Here's how the part is built. I have some questions about the finished solid (model axes, mm). Face numbers are marked on the shaded views. A direction names the side the tool comes from. Round coordinates to 2 decimals unless told otherwise and drop trailing zeros. Write each loop counter-clockwise with the first axis right and the second up, starting at its lowest first coordinate (ties: lowest second). Pieces come first, ordered by that corner, then holes. Notation, with made-up numbers: (87.25, 33) - (132.25, 33) arc R25 cw to (132.25, 50) - close; hole circle Ø3 at (88.5, 85.25). An arc over 180 degrees is marked (long way). One line per item, written item: value. Start each with the question number.
Item 1: Imagine slicing it at D-D, the plane x = 2. Please give me the cut outline in (y, z), then the cut area to 3 significant figures.
Item 2: Imagine slicing it at A-A, the plane z = 1.75. Count the separate pieces of the cut face and the enclosed holes in it, then the cut area to 3 significant figures.
Item 3: For the marked faces 5 and 6, which set-ups out of +Z, -Z, +X, -X, +Y, -Y let a thin tool reach every point of the face, with its end or its side?
Item 4: For P1, Ø4, axis at y = -6, z = 2.5, coming from the -X side; P2, Ø3.5, axis at x = 8.5, y = -1, coming from the -Z side, each with a flat end and sliding along its axis, tell me the tip position at first contact or that it passes through.
Item 5: Imagine slicing it at B-B, the plane x = 40. Please give me the cut outline in (y, z).
Item 6: Imagine slicing it at C-C, the plane x = -26.75. Please give me the cut outline in (y, z), then the cut area to 3 significant figures.
Item 7: Thinking about a two-plate mould opening in X: for the marked faces 1, 2, 3 and 4, which applies, released by +X, released by -X, zero draft, split by the parting line, or undercut?
Item 8: If I drill on line 1 (Y direction, x = -26.75, z = -1); line 2 (Y direction, x = 20, z = 1); line 3 (Y direction, x = 0, z = 1.25), over which ranges is the centre line in solid material (lowest first)?
```python
from build123d import *

# Parameters (mm, degrees)
F0_W        = 60
F0_H        = 15
F0_R        = 1.5
F0_W_2      = 40
F0_R_2      = 1.75
F1_DEPTH    = 5
F2_T        = -2
F3_R        = 5
F4_R        = 5
F5_T1_DEPTH = 100
F5_T3_DEPTH = 5
F5_T6_ANGLE = 90
F5_T8_ANGLE = 90


# Not quite as in the source:
# - a fillet or chamfer that OpenCascade refuses, or shapes differently, is made with other operations: its cross-section is extruded or revolved along the edge and cut away or added


with BuildPart() as f1:
    # F0 (on Top) → F1 (new body, symmetric)
    with BuildSketch(Plane.XY):
        with Locations((-20, 0)):
            Rectangle(F0_W, F0_H)
        with Locations((-45.75, 0)):
            Circle(F0_R, mode=Mode.SUBTRACT)
        with Locations((-26.75, 0)):
            Circle(F0_R, mode=Mode.SUBTRACT)
        with Locations((30, 0)):
            Rectangle(F0_W_2, F0_H)
        with Locations((20, 0)):
            Circle(F0_R_2, mode=Mode.SUBTRACT)
        with Locations((40, 0)):
            Circle(F0_R_2, mode=Mode.SUBTRACT)
    extrude(amount=F1_DEPTH, both=True)

    # F2
    f2_openings = [f1.faces().sort_by_distance(p)[0] for p in [
        (-0.04418, 0, -5),
    ]]
    offset(amount=F2_T, openings=f2_openings, kind=Kind.INTERSECTION)

    # F3
    f3_edges = [f1.edges().sort_by_distance(p)[0] for p in [
        (-50, -7.5, 0),
    ]]
    fillet(f3_edges, radius=F3_R)

    # F4
    f4_edges = [f1.edges().sort_by_distance(p)[0] for p in [
        (-50, 7.5, 0),
    ]]
    fillet(f4_edges, radius=F4_R)

    # F5: fillet of radius 2 on 1 edges, made by hand

    # F5_s2 → F5_t1 (cut)
    with BuildSketch(Plane.YZ.offset(-45)):
        with BuildLine():
            ThreePointArc((-5.5, -5), (-6.9142135624, -4.4142135624), (-7.5, -3))
            Line((-7.5, -3), (-7.5, -5))
            Line((-7.5, -5), (-5.5, -5))
        make_face()
        with BuildLine():
            ThreePointArc((5.5, -5), (6.9142135624, -4.4142135624), (7.5, -3))
            Line((7.5, -3), (7.5, -5))
            Line((7.5, -5), (5.5, -5))
        make_face()
    extrude(amount=F5_T1_DEPTH, mode=Mode.SUBTRACT)

    # F5_s4 → F5_t3 (cut)
    with BuildSketch(Plane.XZ.offset(-2.5)):
        with BuildLine():
            ThreePointArc((-50, -3), (-49.4142135624, -4.4142135624), (-48, -5))
            Line((-48, -5), (-50, -5))
            Line((-50, -5), (-50, -3))
        make_face()
    extrude(amount=F5_T3_DEPTH, mode=Mode.SUBTRACT)

    # F5_s5 → F5_t6 (revolve, cut)
    with BuildSketch(Plane.XZ.offset(2.5)):
        with BuildLine():
            ThreePointArc((-48, -5), (-49.4142135624, -4.4142135624), (-50, -3))
            Line((-50, -3), (-50, -5))
            Line((-50, -5), (-48, -5))
        make_face()
    revolve(axis=Axis((-45, -2.5, -5), (0, 0, 1)), revolution_arc=F5_T6_ANGLE, mode=Mode.SUBTRACT)

    # F5_s7 → F5_t8 (revolve, cut)
    with BuildSketch(Plane.XZ.offset(-2.5)):
        with BuildLine():
            ThreePointArc((-48, -5), (-49.4142135624, -4.4142135624), (-50, -3))
            Line((-50, -3), (-50, -5))
            Line((-50, -5), (-48, -5))
        make_face()
    revolve(axis=Axis((-45, 2.5, -5), (0, 0, -1)), revolution_arc=F5_T8_ANGLE, mode=Mode.SUBTRACT)


with BuildPart() as f6_1:
    # F6: copy of F1
    add(f1.part)


solid = f6_1.part
```
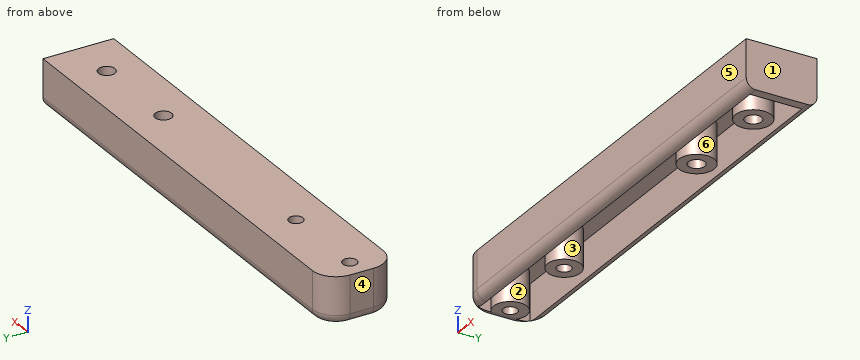
Values follow:
1. outline: (-7.5, -3) arc R2 ccw to (-5.5, -5) - (-5.5, 3) - (5.5, 3) - (5.5, -5) arc R2 ccw to (7.5, -3) - (7.5, 5) - (-7.5, 5) - close
1. area: 60.3 mm^2
2. separate pieces: 4
2. enclosed holes: 5
2. area: 561 mm^2
3. face 5: +Z, -Z, +X, -X, -Y
3. face 6: -Z
4. P1: stops at x = -49.77
4. P2: stops at z = 3
5. outline: (-7.5, -3) arc R2 ccw to (-5.5, -5) - (-5.5, 3) - (-3.75, 3) - (-3.75, -5) - (-1.75, -5) - (-1.75, 5) - (-7.5, 5) - close; (1.75, -5) - (3.75, -5) - (3.75, 3) - (5.5, 3) - (5.5, -5) arc R2 ccw to (7.5, -3) - (7.5, 5) - (1.75, 5) - close
6. outline: (-7.5, -3) arc R2 ccw to (-5.5, -5) - (-5.5, 3) - (-3.5, 3) - (-3.5, -5) - (-1.5, -5) - (-1.5, 5) - (-7.5, 5) - close; (1.5, -5) - (3.5, -5) - (3.5, 3) - (5.5, 3) - (5.5, -5) arc R2 ccw to (7.5, -3) - (7.5, 5) - (1.5, 5) - close
6. area: 86.3 mm^2
7. face 1: released by +X
7. face 2: undercut
7. face 3: undercut
7. face 4: released by -X
8. line 1: y = -7.5 to -5.5, -3.5 to -1.5, 1.5 to 3.5, 5.5 to 7.5
8. line 2: y = -7.5 to -5.5, -3.75 to -1.75, 1.75 to 3.75, 5.5 to 7.5
8. line 3: y = -7.5 to -5.5, 5.5 to 7.5
